Job drawing, mm, ordinate dimensions from the low corner. One solid piece. A direction names the side the tool comes from. Give positions to 0.01 mm unless a question says otherwise; leave off trailing zeros. Loops run counter-clockwise (first coordinate to the right, second up) from the corner with the lowest first, then second, coordinate; pieces in that order, holes last. Notation, with made-up numbers: (54, 43) - (77, 43) arc R32 ccw to (77, 75) - close; hole circle Ø5 at (80, 16.25). An arc over 180 degrees is marked (long way). Answer as CSV lines item,"result". Start each with the question number.
Item 1: Saw through at D-D on x = 16. Give the cut face in (y, z), plus the area to 3 significant figures.
Item 2: Drill centre lines: L1, parallel to Z at x = 5.65, y = 22.85; L2, parallel to Y at x = 11.5, z = 29; L3, parallel to X at y = 22, z = 36. Where is each one in solid material? Low to high. Write a range as from..to.
Item 3: Tool access for the marked faces 1 and 2: list every direction of +Z, -Z, +X, -X, +Y, -Y with a clear straight run to the whole face (end or side of a thin tool).
Item 4: Saw through at C-C on y = 36. Give the cut face in (x, z), plus the area to 3 significant figures.
Item 5: Pin check, flat tips, straight feed: pin 1 (1.5 mm diameter, centred on x = 36, z = 36.5, fed in from -Y); pin 2 (3 mm diameter, centred on x = 5, z = 4.5, fed in from -Y); pin 3 (8 mm diameter, centred on x = 18.5, z = 13.5, fed in from -Y); pin 4 (12 mm diameter, centred on y = 12, z = 33.5, fed in from -X). Stop position of each tip, or through.
Item 6: Saw through at A-A on x = 36.65. Give the cut face in (y, z), plus the area to 3 significant figures.
Item 7: Saw through at B-B on z = 21.15. Give the cut face in (x, y), plus the area to 3 significant figures.
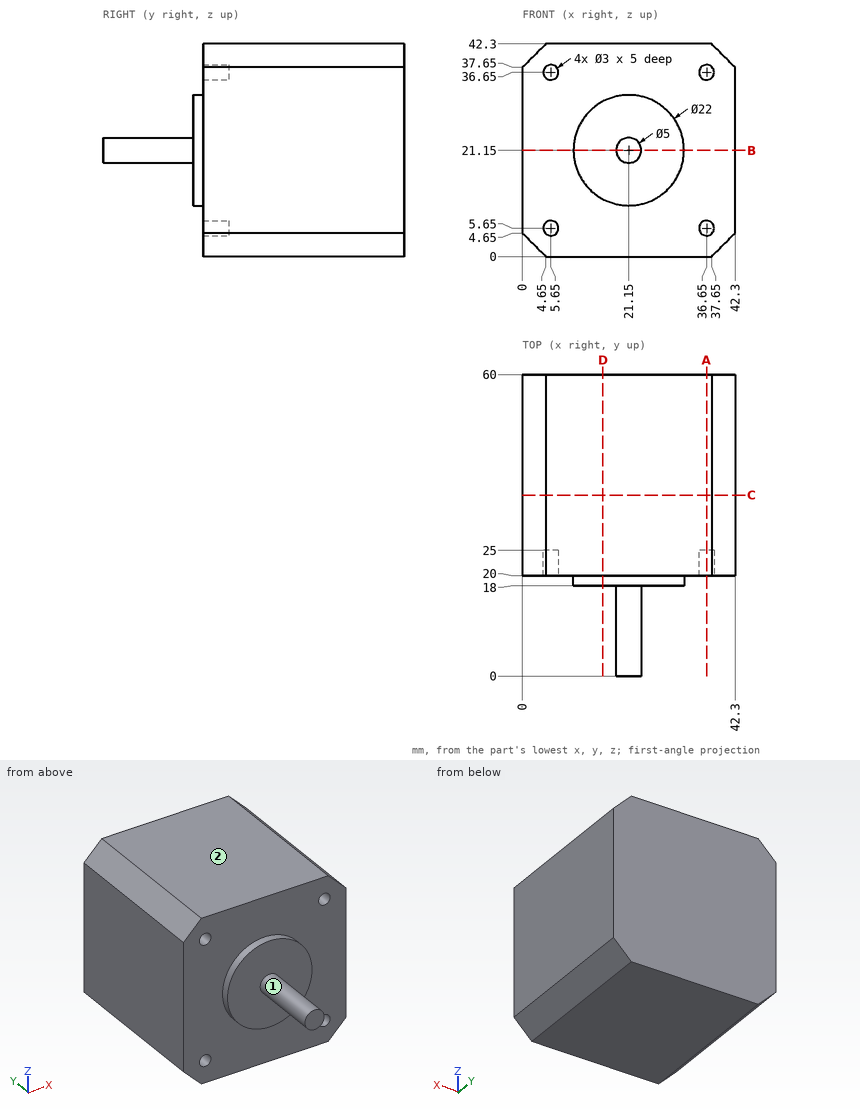
Responses:
1,outline,"(18, 11.43) - (20, 11.43) - (20, 0) - (60, 0) - (60, 42.3) - (20, 42.3) - (20, 30.87) - (18, 30.87) - close"
1,area,"1,730 mm2"
2,L1,"0..4.15, 7.15..35.15, 38.15..42.3"
2,L2,"20..60"
2,L3,"0..4.3, 7..35.3, 38..42.3"
3,face 1,"-Y"
3,face 2,"+Z, +X, -X, +Y, -Y"
4,outline,"(0, 4.65) - (4.65, 0) - (37.65, 0) - (42.3, 4.65) - (42.3, 37.65) - (37.65, 42.3) - (4.65, 42.3) - (0, 37.65) - close"
4,area,"1,750 mm2"
5,pin 1,"y = 25"
5,pin 2,"y = 20"
5,pin 3,"y = 18"
5,pin 4,"through"
6,outline,"(20, 0) - (60, 0) - (60, 42.3) - (20, 42.3) - (20, 38.15) - (25, 38.15) - (25, 35.15) - (20, 35.15) - (20, 7.15) - (25, 7.15) - (25, 4.15) - (20, 4.15) - close"
6,area,"1,660 mm2"
7,outline,"(0, 20) - (10.15, 20) - (10.15, 18) - (18.65, 18) - (18.65, 0) - (23.65, 0) - (23.65, 18) - (32.15, 18) - (32.15, 20) - (42.3, 20) - (42.3, 60) - (0, 60) - close"
7,area,"1,830 mm2"
